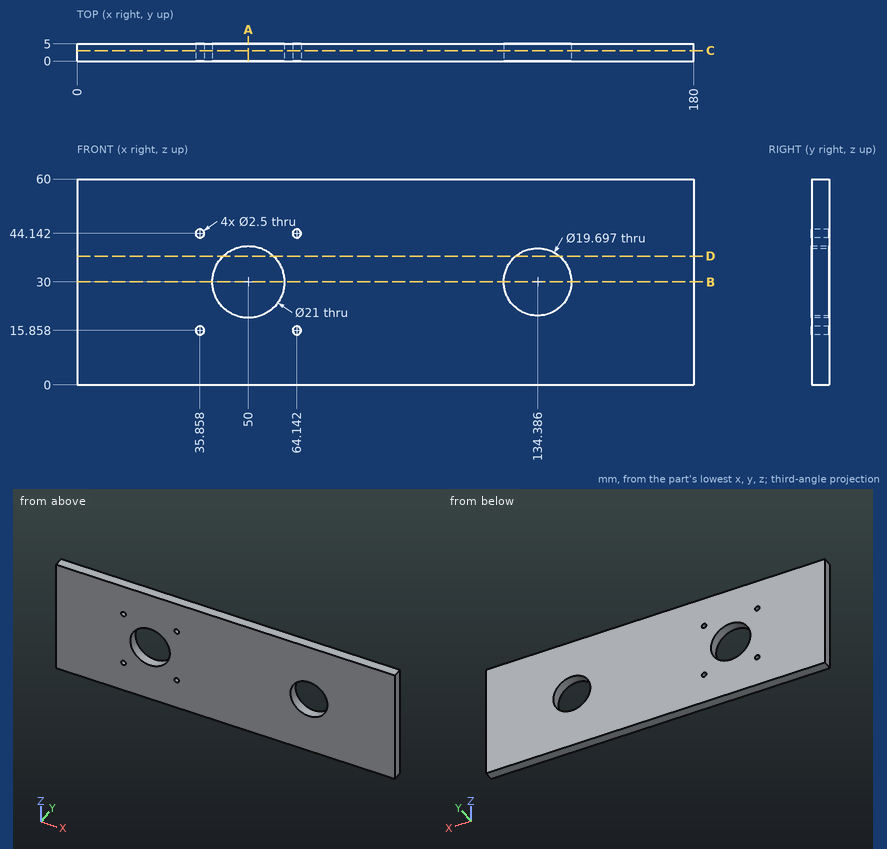
Source: three-view drawing plus pictorial views. Frame: mm from the lowest corner of the part. Coordinates: 2 decimals unless noted, no trailing zeros. Order: outer loops, then holes, each group sorted by start corner. A loop starts at its lowest first (then second) coordinate and runs counter-clockwise, first axis right, second up. Notation, with made-up numbers: M 82,6.25 L 99,6.25 A7 ccw 99,17.25 Z; hole C 88,49.25 d3. An arc over 180 degrees is marked long. One line per question, with ' | ' between items. Start each with the question number.
Item 1: Ray query, probe 1 along X at (y, z) = (1.45, 30.5); probe 2 along Z at (x, y) = (36, 3.5) (1 decimal); probe 3 along X at (y, z) = (4, 27) (1 decimal). Return the intervals inside material, ascending. Write a range as [from, to].
Item 2: Cut plane D-D, the plane z = 37.5. Return the cut outline in (x, y).
Item 3: Pin query (flat end, axial travel): pin 1 Ø2 at (x, z) = (35.86, 44.14) entering from -Y. Return the tip coordinate at first contact, or that it passes through.
Item 4: Cut plane B-B, the plane z = 30. Return the cut outline in (x, y).
Item 5: Cut plane C-C, the plane y = 3.1. Count the separate pieces of the cut face and the enclosed holes in it, then the cut area to 3 significant figures.
Item 6: Cut plane A-A, the plane x = 50. Return the cut outline in (y, z).
A:
1) probe 1: x = [0, 39.51], [60.49, 124.55], [144.22, 180] | probe 2: z = [0, 14.6], [17.1, 42.9], [45.4, 60] | probe 3: x = [0, 39.9], [60.1, 125], [143.8, 180]
2) outline: M 0,0 L 42.65,0 L 42.65,5 L 0,5 Z; M 57.35,0 L 128,0 L 128,5 L 57.35,5 Z; M 140.77,0 L 180,0 L 180,5 L 140.77,5 Z
3) pin 1: passes through
4) outline: M 0,0 L 39.5,0 L 39.5,5 L 0,5 Z; M 60.5,0 L 124.54,0 L 124.54,5 L 60.5,5 Z; M 144.23,0 L 180,0 L 180,5 L 144.23,5 Z
5) separate pieces: 1 | enclosed holes: 6 | area: 10,100 mm2
6) outline: M 0,0 L 5,0 L 5,19.5 L 0,19.5 Z; M 0,40.5 L 5,40.5 L 5,60 L 0,60 Z
